from build123d import *

# Parameters (mm, degrees)
F0_W     = 28
F0_H     = 14
F1_DEPTH = 52
F2_R     = 3
F3_R     = 3


with BuildPart() as f1:
    # F0 (on Front) → F1 (new body)
    with BuildSketch(Plane.XZ):
        Rectangle(F0_W, F0_H)
        with BuildLine():
            Line((14, 7), (14, -7))
            Line((14, -7), (21, -7))
            Line((21, -7), (21, -3))
            ThreePointArc((21, -3), (20.1032778079, 3.8222944655), (14, 7))
        make_face()
        with BuildLine():
            Line((-21, -7), (-14, -7))
            Line((-14, -7), (-14, 7))
            ThreePointArc((-14, 7), (-20.1032778079, 3.8222944655), (-21, -3))
            Line((-21, -3), (-21, -7))
        make_face()
    extrude(amount=F1_DEPTH)

    # F2
    f2_edges = [f1.edges().sort_by_distance(p)[0] for p in [
        (21, -52, -5),
        (20.103278, -52, 3.822294),
        (0, -52, 7),
        (-20.103278, -52, 3.822294),
        (-21, -52, -5),
        (0, -52, -7),
    ]]
    fillet(f2_edges, radius=F2_R)

    # F3
    f3_edges = [f1.edges().sort_by_distance(p)[0] for p in [
        (21, 0, -5),
        (20.103278, 0, 3.822294),
        (0, 0, 7),
        (-20.103278, 0, 3.822294),
        (-21, 0, -5),
        (0, 0, -7),
    ]]
    fillet(f3_edges, radius=F3_R)


solid = f1.part
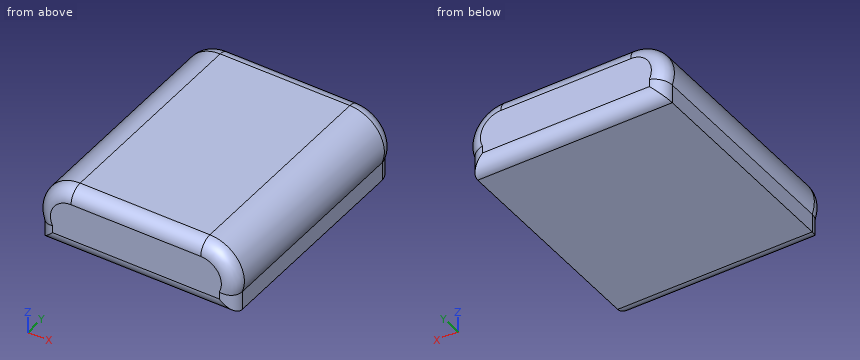
The listing builds one solid part. Answer for the finished solid, in the listing's coordinates (mm). Coordinates: 2 decimals unless noted, no trailing zeros. Loops run counter-clockwise (first coordinate to the right, second up) from the corner with the lowest first, then second, coordinate; pieces in that order, holes last. Notation, with made-up numbers: (86.25, 4.5) -> (113.25, 4.5) arc R28 ccw to (113.25, 40.5) -> close; hole circle Ø10 at (53.5, -1.5). An arc over 180 degrees is marked (long way). Write item = value, one per line. Start each with the question number.
1) A cutting plane is placed at B-B (z = -6). Give the vertices of the cut face in (x, y), then the cut area to 3 significant figures.
2) Given pin 1 Ø4.5 at (y, z) = (-23, -5) entering from -X; pin 2 Ø2 at (y, z) = (-27, -5.5) entering from +X; pin 3 Ø2 at (y, z) = (-7.5, 4) entering from +X, each flat-ended and moving along its own axis, determine where each tip first touches the part or whether it passes through.
3) Straight lines are drawn through the part: line 1 (X direction, y = -37.5, z = -4); line 2 (X direction, y = -46.5, z = -0.25); line 3 (Y direction, x = -3, z = 5.5). For each, find the intervals that lie inside material, in ascending order. Write a range as from..to.
4) A cutting plane is placed at A-A (y = -20). Give the vertices of the cut face in (x, z), then the cut area to 3 significant figures.
Responses:
q1.outline = (-21, -49) arc R3 ccw to (-20, -51.24) -> (20, -51.24) arc R3 ccw to (21, -49) -> (21, -3) arc R3 ccw to (20, -0.76) -> (-20, -0.76) arc R3 ccw to (-21, -3) -> close
q1.area = 2,120 mm²
q2.pin_1 = -21.09
q2.pin_2 = 21
q2.pin_3 = 20.6
q3.line_1 = -21..21
q3.line_2 = -21.45..21.45
q3.line_3 = -51.6..-0.4
q4.outline = (-21, -7) -> (21, -7) -> (21, -3) arc R7.45 ccw to (14, 7) -> (-14, 7) arc R7.45 ccw to (-21, -3) -> close
q4.area = 572 mm²
